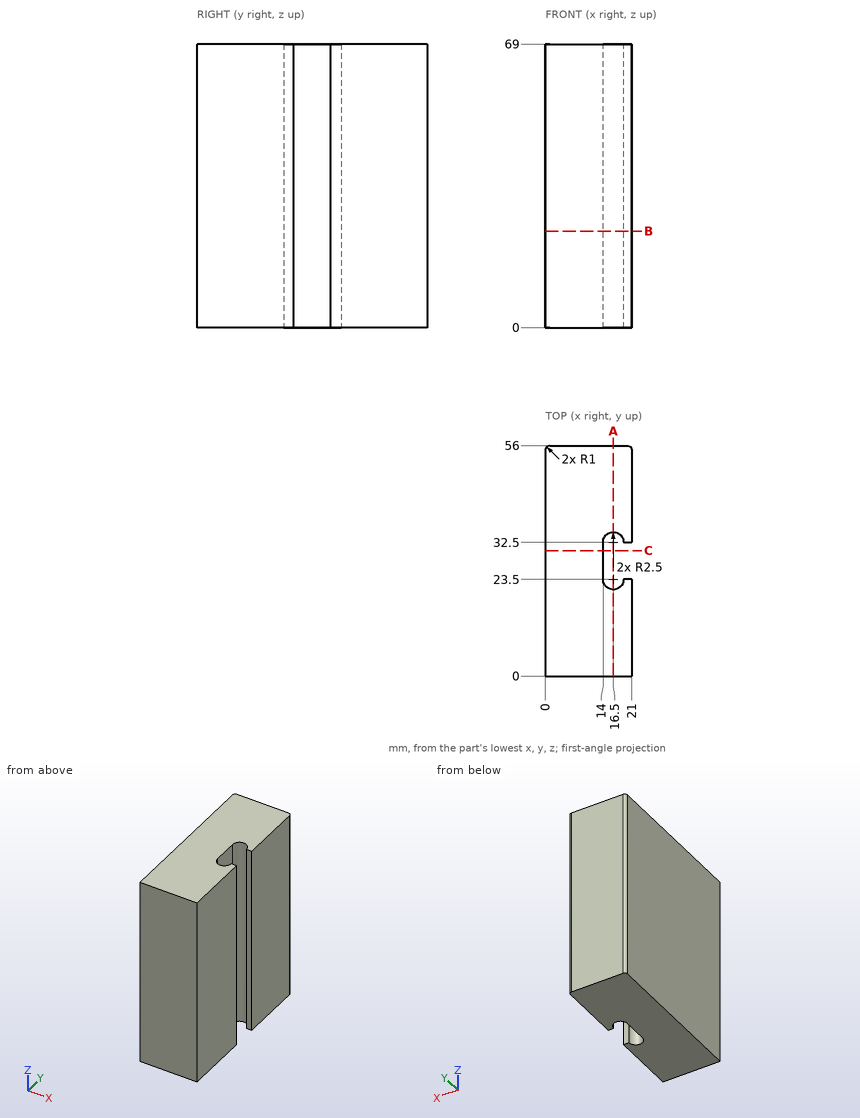
Print and shaded views of the part. All mm, measured from the part's lowest x, y and z. Give positions to 0.01 mm unless a question says otherwise; leave off trailing zeros. Write each loop counter-clockwise with the first axis right and the second up, starting at its lowest first coordinate (ties: lowest second). Pieces come first, ordered by that corner, then holes. Notation, with made-up numbers: M 1.5,-15 L 9.5,-15 A36 cw 9.5,21 Z; hole C -36,23.25 d9. An arc over 180 degrees is marked long. Use a Markdown table: item, result.
1) Cut at A-A (x = 16.5). List the corners of the cut face in (y, z).
Responses:
| item | result |
|---|---|
| outline | M 0,0 L 21,0 L 21,69 L 0,69 Z; M 35,0 L 56,0 L 56,69 L 35,69 Z |
2) Cut at C-C (y = 30.5). List the corners of the cut face in (x, z).
Responses:
| item | result |
|---|---|
| outline | M 0,0 L 14,0 L 14,69 L 0,69 Z |
3) Cut at B-B (z = 23.5). List the corners of the cut face in (x, y), and give its area (3 significant figures).
Responses:
| item | result |
|---|---|
| outline | M 0,0 L 21,0 L 21,23.5 L 19,23.5 A2.5 cw 14,23.5 L 14,32.5 A2.5 cw 19,32.5 L 21,32.5 L 21,55 A1 ccw 20,56 L 1,56 A1 ccw 0,55 Z |
| area | 1,090 mm2 |
4) Drill centre lines: line 1 (X direction, y = 26.5, z = 43.5); line 2 (Y direction, x = 15.75, z = 3.5); line 3 (X direction, y = 21.5, z = 63). Where is each one in solid material? Low to high. Write a range as from..to.
Responses:
| item | result |
|---|---|
| line 1 | x = 0..14 |
| line 2 | y = 0..21.12, 34.88..56 |
| line 3 | x = 0..15, 18..21 |
